Can you work these out from the drawing? Everything is in mm from the part's minimum corner. A direction names the side the tool comes from. Coordinates: 2 decimals unless noted, no trailing zeros. Order: outer loops, then holes, each group sorted by start corner. A loop starts at its lowest first (then second) coordinate and runs counter-clockwise, first axis right, second up. Notation, with made-up numbers: M 36,-16.5 L 69,-16.5 A26 cw 69,10.5 Z; hole C -14.5,32 d9. An arc over 180 degrees is marked long. One line per question, with ' | ' between items. Start each with the question number.
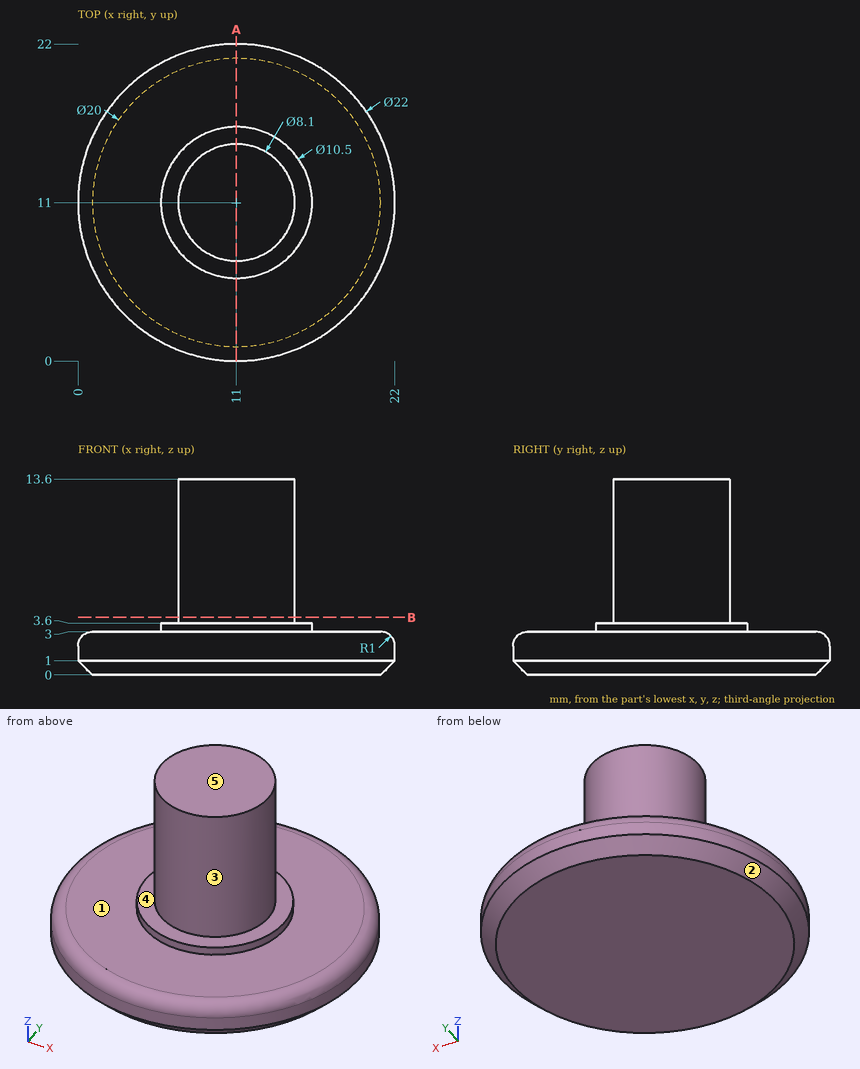
(1) Imagine slicing it at B-B, the plane z = 4. Write out the boundary of the cut face in (x, y).
(2) For P1, Ø6, axis at y = 18.5, z = 4, coming from the -X side; P2, Ø5, axis at y = 5, z = 2.5, coming from the -X side, each with a flat end and sliding along its axis, tell me the tip position at first contact or that it passes through.
(3) Imagine slicing it at A-A, the plane x = 11. Write out the boundary of the cut face in (y, z), plus the area to 3 significant figures.
(4) On a 3-axis mill with a long thin cutter (end or side, diameter ignored), from which of +Z, -Z, +X, -X, +Y, -Y can I reach the whole of each face in a straight line? I mean the marked faces 4 and 5. Say none if no direction works.
(5) If I drill on line 1 along Z through (x, y) = (16.25, 4.5); line 2 along Y through (x, z) = (13.25, 6.5); line 3 along Y through (x, z) = (7.5, 8.5), over which ranges is the centre line in solid material (lowest first)? Write a range as from..to.
(6) We'd pull the mould along Z, two halves only. Please class the marked faces 1, 2 and 3: +Z half, -Z half, draft (parallel to the pull), parting line (faces both ways), or undercut.
Answers:
1) outline: C 11,11 d8.1
2) P1: x = 1.27 | P2: x = 0.59
3) outline: M 0,1 L 1,0 L 21,0 L 22,1 L 22,2 A1 ccw 21,3 L 16.25,3 L 16.25,3.6 L 15.05,3.6 L 15.05,13.6 L 6.95,13.6 L 6.95,3.6 L 5.75,3.6 L 5.75,3 L 1,3 A1 ccw 0,2 Z | area: 152 mm²
4) face 4: +Z | face 5: +Z, +X, -X, +Y, -Y
5) line 1: 0..3 | line 2: 7.63..14.37 | line 3: 8.96..13.04
6) face 1: +Z half | face 2: -Z half | face 3: draft
